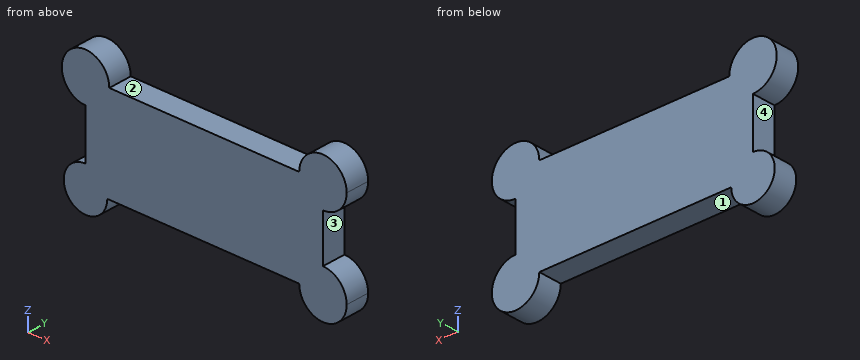
```python
from build123d import *

# Parameters (mm, degrees)
F1_DEPTH = 12.7


with BuildPart() as f1:
    # F0 (on Front) → F1 (new body)
    with BuildSketch(Plane.XZ):
        with BuildLine():
            ThreePointArc((-63.5, 12.7), (-54.5197438789, 16.4197438789), (-50.8, 25.4))
            Line((-50.8, 25.4), (-63.5, 25.4))
            Line((-63.5, 25.4), (-63.5, 12.7))
        make_face()
        with BuildLine():
            Line((-63.5, 25.4), (-50.8, 25.4))
            ThreePointArc((-50.8, 25.4), (-72.4802561211, 34.3802561211), (-63.5, 12.7))
            Line((-63.5, 12.7), (-63.5, 25.4))
        make_face()
        with BuildLine():
            Line((50.8, 25.4), (-50.8, 25.4))
            ThreePointArc((-50.8, 25.4), (-54.5197438789, 16.4197438789), (-63.5, 12.7))
            Line((-63.5, 12.7), (-63.5, -13.7539286115))
            ThreePointArc((-63.5, -13.7539286115), (-55.264983947, -17.164983947), (-51.8539286115, -25.4))
            Line((-51.8539286115, -25.4), (50.8, -25.4))
            ThreePointArc((50.8, -25.4), (54.5197438789, -16.4197438789), (63.5, -12.7))
            Line((63.5, -12.7), (63.5, 12.7))
            ThreePointArc((63.5, 12.7), (54.5197438789, 16.4197438789), (50.8, 25.4))
        make_face()
        with BuildLine():
            ThreePointArc((76.2, 25.4), (63.5, 38.1), (50.8, 25.4))
            Line((50.8, 25.4), (63.5, 25.4))
            Line((63.5, 25.4), (63.5, 12.7))
            ThreePointArc((63.5, 12.7), (72.4802561211, 16.4197438789), (76.2, 25.4))
        make_face()
        with BuildLine():
            Line((63.5, 25.4), (50.8, 25.4))
            ThreePointArc((50.8, 25.4), (54.5197438789, 16.4197438789), (63.5, 12.7))
            Line((63.5, 12.7), (63.5, 25.4))
        make_face()
        with BuildLine():
            ThreePointArc((-51.8539286115, -25.4), (-55.264983947, -17.164983947), (-63.5, -13.7539286115))
            Line((-63.5, -13.7539286115), (-63.5, -25.4))
            Line((-63.5, -25.4), (-51.8539286115, -25.4))
        make_face()
        with BuildLine():
            Line((-63.5, -25.4), (-63.5, -13.7539286115))
            ThreePointArc((-63.5, -13.7539286115), (-71.735016053, -33.635016053), (-51.8539286115, -25.4))
            Line((-51.8539286115, -25.4), (-63.5, -25.4))
        make_face()
        with BuildLine():
            ThreePointArc((76.2, -25.4), (72.4802561211, -16.4197438789), (63.5, -12.7))
            Line((63.5, -12.7), (63.5, -25.4))
            Line((63.5, -25.4), (50.8, -25.4))
            ThreePointArc((50.8, -25.4), (63.5, -38.1), (76.2, -25.4))
        make_face()
        with BuildLine():
            Line((63.5, -25.4), (63.5, -12.7))
            ThreePointArc((63.5, -12.7), (54.5197438789, -16.4197438789), (50.8, -25.4))
            Line((50.8, -25.4), (63.5, -25.4))
        make_face()
    extrude(amount=F1_DEPTH)


solid = f1.part
```
CAD build for the part. Positions are in the model's coordinates, mm. Face numbers are marked on the shaded views. Round coordinates to 2 decimals unless told otherwise and drop trailing zeros. Order: outer loops, then holes, each group sorted by start corner. A loop starts at its lowest first (then second) coordinate and runs counter-clockwise, first axis right, second up. Notation, with made-up numbers: (-36, 46.5) -> (-27, 46.5) arc R17 cw to (-27, 70.5) -> close; hole circle Ø3 at (86, 45). An arc over 180 degrees is marked (long way). One line per question, with ' | ' between items.
Q1. Drop flat-ended pins along their axis: pin 1 (10 mm diameter, centred on x = -7.5, z = 27.5, fed in from -Y); pin 2 (4 mm diameter, centred on x = 22.5, y = -8.5, fed in from -Z); pin 3 (5 mm diameter, centred on y = -4, z = -14.5, fed in from +X); pin 4 (4 mm diameter, centred on y = -5, z = 0, fed in from +X). Give the stop position or say it passes through.
Completed:
pin 1: stops at y = -12.7 | pin 2: stops at z = -25.4 | pin 3: stops at x = 73.03 | pin 4: stops at x = 63.5
Q2. Slice it at A-A (y = -6.25). Write the cut outline in (x, z), then the cut area to 3 significant figures.
Completed:
outline: (-63.5, -13.75) arc R11.65 ccw (long way) to (-51.85, -25.4) -> (50.8, -25.4) arc R12.7 ccw (long way) to (63.5, -12.7) -> (63.5, 12.7) arc R12.7 ccw (long way) to (50.8, 25.4) -> (-50.8, 25.4) arc R12.7 ccw (long way) to (-63.5, 12.7) -> close | area: 7,910 mm^2
Q3. Two-plate mould, pull along X, no slides. Class the marked faces 1, 2, 3 and 4: released by +X, released by -X, zero draft, split by the parting line, or undercut.
Completed:
face 1: undercut | face 2: undercut | face 3: released by +X | face 4: released by -X
Q4. Probe probe 1 along Z at (x, y) = (-20, -0.75); probe 2 along X at (y, z) = (-2.5, 35); probe 3 along X at (y, z) = (-8.5, -25.5). List the from-to ranges inside material, lowest first.
Completed:
probe 1: z = -25.4 to 25.4 | probe 2: x = -71.81 to -55.19, 55.19 to 71.81 | probe 3: x = -75.15 to -51.85, 50.8 to 76.2
Q5. Slice it at B-B (x = 12.5). Write the cut outline in (y, z).
Completed:
outline: (-12.7, -25.4) -> (0, -25.4) -> (0, 25.4) -> (-12.7, 25.4) -> close
Q6. Slice it at C-C (z = 9). Write the cut outline in (x, y), then the cut area to 3 significant figures.
Completed:
outline: (-63.5, -12.7) -> (63.5, -12.7) -> (63.5, 0) -> (-63.5, 0) -> close | area: 1,610 mm^2
